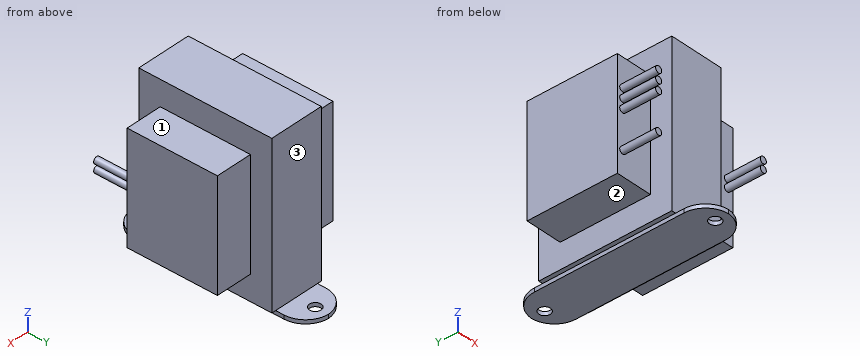
from build123d import *

# Parameters (mm, degrees)
F0_W         = 19.3
F0_H         = 82.5
F1_DEPTH     = 1.6
F2_W         = 22.8
F2_H         = 55.6
F3_DEPTH     = 66.7
F4_W         = 37.7
F4_H         = 45.7
F5_DEPTH     = 15.25
F6_W         = 37.7
F6_H         = 45.7
F7_DEPTH     = 15.25
F8_R         = 2.4
F9_DEPTH     = 68.301
F10_T1_DEPTH = 51.6
F11_R        = 1.4
F12_DEPTH    = 15
F13_R        = 1.4
F14_DEPTH    = 15


# Not quite as in the source:
# - a fillet or chamfer that OpenCascade refuses, or shapes differently, is made with other operations: its cross-section is extruded or revolved along the edge and cut away or added


with BuildPart() as f1:
    # F0 (on Top) → F1 (new body)
    with BuildSketch(Plane.XY):
        Rectangle(F0_W, F0_H)
    extrude(amount=F1_DEPTH)

    # F2 (on face) → F3 (join)
    with BuildSketch(Plane.XY.offset(1.6)):
        Rectangle(F2_W, F2_H)
    extrude(amount=F3_DEPTH)

    # F4 (on face) → F5 (join)
    with BuildSketch(Plane(origin=(-11.4, 0, 0), x_dir=(0, -1, 0), z_dir=(-1, 0, 0))):
        with Locations((0, 34.95)):
            Rectangle(F4_W, F4_H)
    extrude(amount=F5_DEPTH)

    # F6 (on face) → F7 (join)
    with BuildSketch(Plane.YZ.offset(11.4)):
        with Locations((0, 34.95)):
            Rectangle(F6_W, F6_H)
    extrude(amount=F7_DEPTH)

    # F8 (on face) → F9 (cut, through all)
    with BuildSketch(Plane(origin=(0, 0, 0), x_dir=(1, 0, 0), z_dir=(0, 0, -1))):
        with Locations((0, 35.65)):
            Circle(F8_R)
        with Locations((0, -35.65)):
            Circle(F8_R)
    extrude(amount=-F9_DEPTH, mode=Mode.SUBTRACT)

    # F10: fillet of radius 10 on 4 edges, made by hand

    # F10_s2 → F10_t1 (cut)
    with BuildSketch(Plane.XY.offset(-25)):
        with BuildLine():
            ThreePointArc((0.35, 41.25), (-6.7210678119, 38.3210678119), (-9.65, 31.25))
            Line((-9.65, 31.25), (-9.65, 41.25))
            Line((-9.65, 41.25), (0.35, 41.25))
        make_face()
        with BuildLine():
            ThreePointArc((9.65, 31.25), (6.7210678119, 38.3210678119), (-0.35, 41.25))
            Line((-0.35, 41.25), (9.65, 41.25))
            Line((9.65, 41.25), (9.65, 31.25))
        make_face()
        with BuildLine():
            ThreePointArc((9.65, -31.25), (6.7210678119, -38.3210678119), (-0.35, -41.25))
            Line((-0.35, -41.25), (9.65, -41.25))
            Line((9.65, -41.25), (9.65, -31.25))
        make_face()
        with BuildLine():
            ThreePointArc((0.35, -41.25), (-6.7210678119, -38.3210678119), (-9.65, -31.25))
            Line((-9.65, -31.25), (-9.65, -41.25))
            Line((-9.65, -41.25), (0.35, -41.25))
        make_face()
    extrude(amount=F10_T1_DEPTH, mode=Mode.SUBTRACT)

    # F11 (on face) → F12 (join)
    with BuildSketch(Plane.XZ.offset(18.85)):
        with Locations((-24.15, 41.8)):
            Circle(F11_R)
        with Locations((-24.15, 45.8)):
            Circle(F11_R)
        with Locations((-24.15, 37.8)):
            Circle(F11_R)
        with Locations((-24.15, 22.1)):
            Circle(F11_R)
    extrude(amount=F12_DEPTH)

    # F13 (on face) → F14 (join)
    with BuildSketch(Plane.XZ.offset(18.85)):
        with Locations((24.15, 36.9742031991)):
            Circle(F13_R)
        with Locations((24.15, 33.4742031991)):
            Circle(F13_R)
    extrude(amount=F14_DEPTH)


solid = f1.part
Geometry: final body of the model. Coordinates: model frame, mm. Face numbers are marked on the shaded views. A direction names the side the tool comes from. Give positions to 0.01 mm unless a question says otherwise; leave off trailing zeros. Write each loop counter-clockwise with the first axis right and the second up, starting at its lowest first coordinate (ties: lowest second). Pieces come first, ordered by that corner, then holes.
(1) Cut plane C-C, the plane x = 24.15. Return loops of the section in (y, z).
(2) Ray query, line 1 (Y direction, x = 0, z = 0.55); line 2 (Y direction, x = 1, z = 51.5); line 3 (Y direction, x = -23, z = 17.5). Return the intervals inside material, ascending.
(3) Access query for the marked faces 1, 2 and 3. Directions: +Z, -Z, +X, -X, +Y, -Y. A direction counts if a zero-diameter tool reaches every point of the face in a straight line with its end or side. Return the directions, or none.
(4) First-contact query: P1, Ø2, axis at y = 24.5, z = 45.5, coming from the -X side; P2, Ø5, axis at x = -17, y = -11, coming from the +Z side; P3, Ø3, axis at x = 0, y = -35.65, coming from the -Z side; P4, Ø0.8, axis at x = -23.5, z = 46.5, coming from the -Y side. Flat tips, straight axial feed; report the tip coordinate or a pass-through.
(5) Cut plane A-A, the plane z = 22.1. Return loops of the section in (x, y).
(6) Cut plane D-D, the plane y = 25.5. Return loops of the section in (x, z).
(7) Cut plane B-B, the plane y = 35.65. Return loops of the section in (x, z).
Values follow:
1. outline: (-33.85, 32.07) - (-18.85, 32.07) - (-18.85, 12.1) - (18.85, 12.1) - (18.85, 57.8) - (-18.85, 57.8) - (-18.85, 38.37) - (-33.85, 38.37) - (-33.85, 35.57) - (-18.85, 35.57) - (-18.85, 34.87) - (-33.85, 34.87) - close
2. line 1: y = -41.24 to -38.05, -33.25 to 33.25, 38.05 to 41.24
2. line 2: y = -27.8 to 27.8
2. line 3: y = -18.85 to 18.85
3. face 1: +Z, +X, +Y, -Y
3. face 2: -Z, -X, +Y, -Y
3. face 3: +Z, +X, -X, +Y
4. P1: stops at x = -11.4
4. P2: stops at z = 57.8
4. P3: passes through
4. P4: stops at y = -33.85
5. outline: (-26.65, -18.85) - (-25.55, -18.85) - (-25.55, -33.85) - (-22.75, -33.85) - (-22.75, -18.85) - (-11.4, -18.85) - (-11.4, -27.8) - (11.4, -27.8) - (11.4, -18.85) - (26.65, -18.85) - (26.65, 18.85) - (11.4, 18.85) - (11.4, 27.8) - (-11.4, 27.8) - (-11.4, 18.85) - (-26.65, 18.85) - close
6. outline: (-11.4, 1.6) - (-9.65, 1.6) - (-9.65, 0) - (9.65, 0) - (9.65, 1.6) - (11.4, 1.6) - (11.4, 68.3) - (-11.4, 68.3) - close
7. outline: (-8.63, 0) - (-2.4, 0) - (-2.4, 1.6) - (-8.63, 1.6) - close; (2.4, 0) - (8.63, 0) - (8.63, 1.6) - (2.4, 1.6) - close
